Verification items for the finished model (mm, model axes). A direction names the side the tool comes from. Give positions to 0.01 mm unless a question says otherwise; leave off trailing zeros. Order: outer loops, then holes, each group sorted by start corner. A loop starts at its lowest first (then second) coordinate and runs counter-clockwise, first axis right, second up. Notation, with made-up numbers: (71.5, 28.25) -> (124.5, 28.25) arc R15 cw to (124.5, 48.25) -> close; hole circle Ø1 at (29.5, 78). An arc over 180 degrees is marked (long way). Return JSON: item names as keys, results as strings. Group by question number.
(1) Cross-section at C-C on x = -1.5. Enter the section's corners in (y, z), then the cut area to 3 significant figures.
(2) Cross-section at D-D on y = 3. Enter the section's corners in (x, z).
(3) Depth check by flat-ended pin: pin 1 Ø1 at (x, y) = (0, 7.5) entering from +Z; pin 2 Ø1 at (y, z) = (5.5, 3) entering from +X. Enter the tip coordinate at first touch or a pass-through.
(4) Tool access check on faces 4 (the face through (4.637, 9.549, 1.03)), 5 (the face through (-1.24, 2.84, 4.3)), 6 (the face through (-1.95, 3.04, -6.2)), 7 (the face through (4.3, 2.95, -1.25)). Record the directions out of +Z, -Z, +X, -X, +Y, -Y that give a thin tool (end or side, any length) a straight path to the whole face; none if there is none.
(5) Cross-section at B-B on z = 0. Enter the section's corners in (x, y), then the cut area to 3 significant figures.
(6) Thickness scan on line 1 along X through (y, z) = (7, 0); line 2 along Y through (x, z) = (4.25, 4.25); line 3 along X through (y, z) = (5.5, 0). Record the ranges inside material, lowest first.
(7) Release check for a two-part mould opening along Y. For faces 1 (the face through (0, 0, 3)), 2 (the face through (5, 6, 0)), 3 (the face through (3.955, 13.507, 5.158)) record: pulls with the +Y half, pulls with the -Y half, needs draft (parallel to the pull), parting line crosses it, or undercut.
(8) Cross-section at A-A on x = 0. Enter the section's corners in (y, z), then the cut area to 3 significant figures.
from build123d import *


with BuildPart() as part:
    # 草图1 → 旋转1 (revolve)
    with BuildSketch(Plane.XY, mode=Mode.PRIVATE) as revolve_1_sk:
        Polygon((2.5, 0), (6.5, 0), (6.5, 6), (4.75, 6), (4.75, 13), (6.5, 13), (6.5, 14), (2.5, 14), align=None)
    revolve(revolve_1_sk.sketch.rotate(Axis((0, 0, 0), (0, 1, 0)), 90), axis=Axis((0, 0, 0), (0, 1, 0)))

    # 草图3 → M3 螺纹孔1 (revolve, cut)
    with BuildSketch(Plane(origin=(0, 3, 0), x_dir=(0, 1, 0), z_dir=(1, 0, 0))):
        Polygon((0, 0), (0, 6.5), (1.25, 6.5), (1.25, 0.275), (1.525, 0), align=None)
    revolve(axis=Axis((0, 3, -6.35), (0, 0, 1)), mode=Mode.SUBTRACT)

    # 草图5 → M3 螺纹孔2 (revolve, cut)
    with BuildSketch(Plane.ZX.offset(3)):
        Polygon((0, 0), (0, 6.5), (1.25, 6.5), (1.25, 0.275), (1.525, 0), align=None)
    revolve(axis=Axis((-6.35, 3, 0), (1, 0, 0)), mode=Mode.SUBTRACT)


solid = part.part
Verdict:
{
 "1": {"outline": "(0, -6.32) -> (6, -6.32) -> (6, -4.51) -> (13, -4.51) -> (13, -6.32) -> (14, -6.32) -> (14, -2) -> (0, -2) -> close; (0, 2) -> (14, 2) -> (14, 6.32) -> (13, 6.32) -> (13, 4.51) -> (6, 4.51) -> (6, 6.32) -> (0, 6.32) -> close", "area": "95.6 mm²"},
 "2": {"outline": "(-1.25, 2.17) -> (-1.25, 6.38) arc R6.5 ccw (long way) to (6.38, -1.25) -> (2.17, -1.25) arc R2.5 cw (long way) to start; (1.25, 2.17) arc R2.5 cw to (2.17, 1.25) -> (6.38, 1.25) arc R6.5 ccw to (1.25, 6.38) -> close"},
 "3": {"pin 1": "z = 4.75", "pin 2": "x = 6"},
 "4": {"face 4": "none", "face 5": "+Z", "face 6": "+Y, -Y", "face 7": "+X"},
 "5": {"outline": "(-6.5, 0) -> (-2.5, 0) -> (-2.5, 14) -> (-6.5, 14) -> (-6.5, 13) -> (-4.75, 13) -> (-4.75, 6) -> (-6.5, 6) -> close; (2.5, 0) -> (6.5, 0) -> (6.5, 1.75) -> (2.5, 1.75) -> close; (2.5, 4.25) -> (6.5, 4.25) -> (6.5, 6) -> (4.75, 6) -> (4.75, 13) -> (6.5, 13) -> (6.5, 14) -> (2.5, 14) -> close", "area": "77.5 mm²"},
 "6": {"line 1": "-4.75 to -2.5, 2.5 to 4.75", "line 2": "0 to 6, 13 to 14", "line 3": "-6.5 to -2.5, 2.5 to 6.5"},
 "7": {"face 1": "pulls with the -Y half", "face 2": "undercut", "face 3": "needs draft"},
 "8": {"outline": "(0, -6.5) -> (6, -6.5) -> (6, -4.75) -> (13, -4.75) -> (13, -6.5) -> (14, -6.5) -> (14, -2.5) -> (0, -2.5) -> close; (0, 2.5) -> (1.75, 2.5) -> (1.75, 6.5) -> (0, 6.5) -> close; (4.25, 2.5) -> (14, 2.5) -> (14, 6.5) -> (13, 6.5) -> (13, 4.75) -> (6, 4.75) -> (6, 6.5) -> (4.25, 6.5) -> close", "area": "77.5 mm²"}
}
